```python
from build123d import *

# Parameters (mm, degrees)
CROQUIS1_R                   = 3
SALIENTE_EXTRUIR1_DEPTH      = 18
CROQUIS1_2_R                 = 3
SALIENTE_EXTRUIR2_DEPTH      = 21.5
SALIENTE_EXTRUIR2_DEPTH_BACK = 1.5
CROQUIS3_R                   = 3
CORTAR_EXTRUIR1_DEPTH        = 4
CROQUIS9_R                   = 1.125
SALIENTE_EXTRUIR3_DEPTH      = 55
CROQUIS10_R                  = 0.75
SALIENTE_EXTRUIR4_DEPTH      = 112


with BuildPart() as part:
    # Croquis1 → Saliente-Extruir1 (new body)
    with BuildSketch(Plane.XY):
        Circle(CROQUIS1_R)
    extrude(amount=SALIENTE_EXTRUIR1_DEPTH)

    # Croquis1_2 → Saliente-Extruir2 (add, two sides)
    with BuildSketch(Plane.XY) as saliente_extruir2_sk:
        Circle(CROQUIS1_2_R)
    extrude(amount=SALIENTE_EXTRUIR2_DEPTH)
    extrude(saliente_extruir2_sk.sketch, amount=-SALIENTE_EXTRUIR2_DEPTH_BACK)

    # Croquis3 → Cortar-Extruir1 (cut)
    with BuildSketch(Plane(origin=(0, 0, -1.5), x_dir=(-1, 0, 0), z_dir=(0, 0, -1))):
        Circle(CROQUIS3_R)
    extrude(amount=-CORTAR_EXTRUIR1_DEPTH, mode=Mode.SUBTRACT)

    # Croquis9 → Saliente-Extruir3 (add)
    with BuildSketch(Plane.XY.offset(21.5)):
        with Locations((0, -1.15)):
            Circle(CROQUIS9_R)
        with Locations((0, 1.15)):
            Circle(CROQUIS9_R)
    extrude(amount=SALIENTE_EXTRUIR3_DEPTH)

    # Croquis10 → Saliente-Extruir4 (add)
    with BuildSketch(Plane.XY.offset(21.5)):
        with Locations((0, -1.15)):
            Circle(CROQUIS10_R)
        with Locations((0, 1.15)):
            Circle(CROQUIS10_R)
    extrude(amount=SALIENTE_EXTRUIR4_DEPTH)


solid = part.part
```
The model under review builds one solid part; all positions refer to its coordinate system, in mm. Round coordinates to 2 decimals unless told otherwise and drop trailing zeros. Order: outer loops, then holes, each group sorted by start corner. A loop starts at its lowest first (then second) coordinate and runs counter-clockwise, first axis right, second up. Notation, with made-up numbers: (23, 60.5) - (49, 60.5) arc R22 cw to (49, 76.5) - close; hole circle Ø5 at (-26.5, 63). An arc over 180 degrees is marked (long way). Answer in a Markdown table with one row per item.
(1) Take a section at A-A on z = 117. Write out the cut boundary in (x, y), plus the area to 3 significant figures.
Result set:
| item | result |
|---|---|
| outline | circle Ø1.5 at (0, -1.15); circle Ø1.5 at (0, 1.15) |
| area | 3.53 mm2 |
(2) Take a section at C-C on z = 17.5. Write out the cut boundary in (x, y).
Result set:
| item | result |
|---|---|
| outline | circle Ø6 at (0, 0) |
(3) Clearance check with flat-ended pins moving along their axes: P1, Ø2, axis at y = 0, z = 72.5, coming from the +X side; P2, Ø1, axis at x = 2, y = 2, coming from the +Z side. State where each tip first meets the part, or that it passes through.
Result set:
| item | result |
|---|---|
| P1 | stops at x = 1.11 |
| P2 | stops at z = 21.5 |
(4) For line 1 (X direction, y = -0.4, z = 20.5); line 2 (Z direction, x = 2.6, y = -1.3); line 3 (Z direction, x = 0, y = -2.2), list the stretches that pass through material, from the lowest coordinate up. Write a range as from..to.
Result set:
| item | result |
|---|---|
| line 1 | x = -2.97..2.97 |
| line 2 | z = 2.5..21.5 |
| line 3 | z = 2.5..76.5 |
(5) Take a section at B-B on z = 53. Write out the cut boundary in (x, y) (3 decimals), plus the area to 3 significant figures.
Result set:
| item | result |
|---|---|
| outline | circle Ø2.25 at (0, -1.15); circle Ø2.25 at (0, 1.15) |
| area | 7.95 mm2 |
(6) Mouldability with a two-part tool opening along Y and no side actions: class faces 1 (the face through (0, 0, 2.5)), 2 (the face through (0.6, -0.2, 48.6)), 3 (the face through (-3, 0, 12)) as released by +Y, released by -Y, zero draft, split by the parting line, or undercut.
Result set:
| item | result |
|---|---|
| face 1 | zero draft |
| face 2 | undercut |
| face 3 | split by the parting line |
